Study the drawing (mm; zero at the part's minimum x, y, z) and answer. A direction names the side the tool comes from. Give positions to 0.01 mm unless a question says otherwise; leave off trailing zeros. Order: outer loops, then holes, each group sorted by start corner. A loop starts at its lowest first (then second) coordinate and runs counter-clockwise, first axis right, second up. Notation, with made-up numbers: (31.25, -12) -> (55.25, -12) arc R14 cw to (55.25, 0) -> close; hole circle Ø4 at (40, -35). An arc over 180 degrees is marked (long way). One line per question, with ' | ' between items. Start each with the question number.
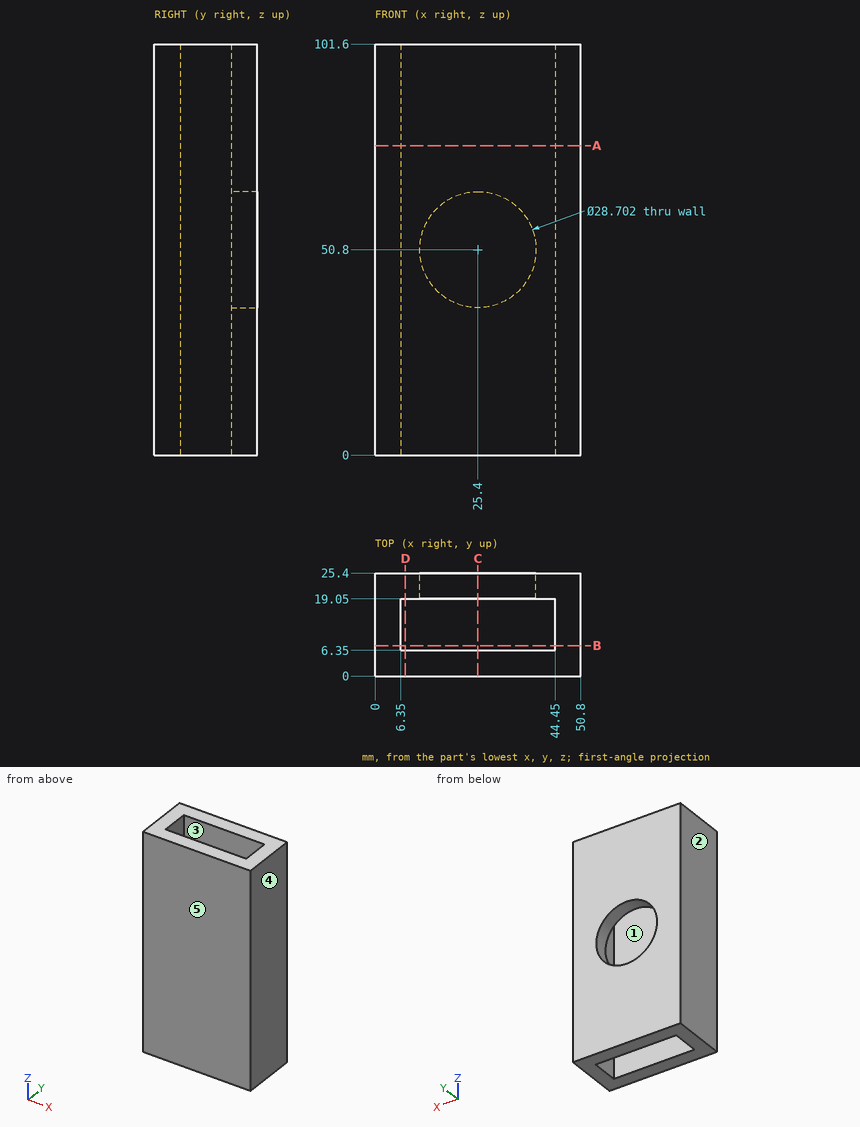
Q1. A cutting plane is placed at A-A, the plane z = 76.5. Determine the outline of the cut face in (x, y).
Q2. A cutting plane is placed at C-C, the plane x = 25.4. Determine the outline of the cut face in (y, z), then the cut area to 3 significant figures.
Q3. A cutting plane is placed at D-D, the plane x = 7.5. Determine the outline of the cut face in (y, z), then the cut area to 3 significant figures.
Q4. Determine the mould class of the marked faces 3, 4 and 5 for opening direction X: pulls with the +X half, pulls with the -X half, needs draft (parallel to the pull), parting line crosses it, or undercut.
Q5. Find the intervals of material crossed by line 1 (X direction, y = 7.5, z = 56.5); line 2 (Y direction, x = 10, z = 15.5); line 3 (X direction, y = 22, z = 50.8), in increasing order.
Q6. Which of the six approach directions +Z, -Z, +X, -X, +Y, -Y give full straight-line access (tool end or side, diameter ignored) to the marked faces 1 and 2?
Q7. A cutting plane is placed at B-B, the plane y = 7.5. Determine the outline of the cut face in (x, z).
Geometry results:
1) outline: (0, 0) -> (50.8, 0) -> (50.8, 25.4) -> (0, 25.4) -> close; hole (6.35, 6.35) -> (44.45, 6.35) -> (44.45, 19.05) -> (6.35, 19.05) -> close
2) outline: (0, 0) -> (6.35, 0) -> (6.35, 101.6) -> (0, 101.6) -> close; (19.05, 0) -> (25.4, 0) -> (25.4, 36.45) -> (19.05, 36.45) -> close; (19.05, 65.15) -> (25.4, 65.15) -> (25.4, 101.6) -> (19.05, 101.6) -> close | area: 1,110 mm²
3) outline: (0, 0) -> (6.35, 0) -> (6.35, 101.6) -> (0, 101.6) -> close; (19.05, 0) -> (25.4, 0) -> (25.4, 101.6) -> (19.05, 101.6) -> close | area: 1,290 mm²
4) face 3: undercut | face 4: pulls with the +X half | face 5: needs draft
5) line 1: 0 to 6.35, 44.45 to 50.8 | line 2: 0 to 6.35, 19.05 to 25.4 | line 3: 0 to 11.05, 39.75 to 50.8
6) face 1: +Z, -Z | face 2: +Z, -Z, -X, +Y, -Y
7) outline: (0, 0) -> (6.35, 0) -> (6.35, 101.6) -> (0, 101.6) -> close; (44.45, 0) -> (50.8, 0) -> (50.8, 101.6) -> (44.45, 101.6) -> close
